Design review of the part built by this model. Coordinates are the model's own, in mm. A direction names the side the tool comes from. Coordinates: 2 decimals unless noted, no trailing zeros. Loops run counter-clockwise (first coordinate to the right, second up) from the corner with the lowest first, then second, coordinate; pieces in that order, holes last. Notation, with made-up numbers: (84.5, 1) -> (94.5, 1) arc R18 ccw to (94.5, 12) -> close; hole circle Ø4 at (-23, -24). An arc over 180 degrees is marked (long way). Use CSV: the item, a comma, the result in double quotes.
```python
from build123d import *

# Parameters (mm, degrees)
CROQUIS1_W              = 44.5
CROQUIS1_H              = 12
CROQUIS1_W_2            = 3
CROQUIS1_H_2            = 7
SALIENTE_EXTRUIR1_DEPTH = 3
EXTRUIR_L_MINA1_DEPTH   = 3


with BuildPart() as part:
    # Croquis1 → Saliente-Extruir1 (new body)
    with BuildSketch(Plane.XY):
        Polygon((-15, -12), (15, -12), (22.25, -6), (-22.25, -6), align=None)
        Rectangle(CROQUIS1_W, CROQUIS1_H)
        Polygon((9, 22), (22.25, 6), (-22.25, 6), (-9, 22), align=None)
        with Locations((23.75, 0)):
            Rectangle(CROQUIS1_W_2, CROQUIS1_H_2)
        with Locations((-23.75, 0)):
            Rectangle(CROQUIS1_W_2, CROQUIS1_H_2)
    extrude(amount=SALIENTE_EXTRUIR1_DEPTH)

    # Croquis2 → Extruir-Lámina1 (add, through all)
    with BuildSketch(Plane.XY.offset(3)):
        Polygon((10.313415418, 68.264367666), (31.70862995, 32.607243184), (0, 0), (-31.70862995, 32.607243184), (-10.313415418, 68.264367666), (-15.458313145, 71.35144191), (-39.229366975, 31.734759205), (0, -8.606356476), (39.229366975, 31.734759205), (15.458313145, 71.35144191), align=None)
    extrude(amount=-EXTRUIR_L_MINA1_DEPTH)


solid = part.part
```
Item 1: Clearance check with flat-ended pins moving along their axes: pin 1 (0.8 mm diameter, centred on y = 5.5, z = 1.5, fed in from +X); pin 2 (1 mm diameter, centred on x = -25, y = 48, fed in from -Z); pin 3 (0.9 mm diameter, centred on y = -0.5, z = 2, fed in from +X); pin 4 (0.8 mm diameter, centred on y = 4, z = 1.5, fed in from -X). State where each tip first meets the part, or that it passes through.
Checked values:
pin 1,"x = 22.25"
pin 2,"z = 0"
pin 3,"x = 25.25"
pin 4,"x = -22.25"
Item 2: Machinability: for faces 1 (the face through (24, 3.5, 1)), 2 (the face through (12.92, 69.83, 1.52)), 3 (the face through (-25.25, 0, 1)), 4 (the face through (11.81, 18.607, 1.479)), 5 (the face through (24, -3.5, 1)), which of the approach directions +Z, -Z, +X, -X, +Y, -Y give a long, thin tool a straight path to every point of the face, cutting with its end or side? Answer none if there is none.
Checked values:
face 1,"+Z, -Z, +X"
face 2,"+Z, -Z, +Y"
face 3,"+Z, -Z, -X, -Y"
face 4,"+Z, -Z"
face 5,"+Z, -Z, +X, -Y"
Item 3: Add section C-C (z = 2.55). Give the boundary of the cut face in (x, y), then the cut area to 3 significant figures.
Checked values:
outline,"(-39.23, 31.73) -> (-18.55, 10.47) -> (-22.25, 6) -> (-22.25, 3.5) -> (-25.25, 3.5) -> (-25.25, -3.5) -> (-22.25, -3.5) -> (-22.25, -6) -> (-15, -12) -> (15, -12) -> (22.25, -6) -> (22.25, -3.5) -> (25.25, -3.5) -> (25.25, 3.5) -> (22.25, 3.5) -> (22.25, 6) -> (18.55, 10.47) -> (39.23, 31.73) -> (15.46, 71.35) -> (10.31, 68.26) -> (31.71, 32.61) -> (14.7, 15.12) -> (9, 22) -> (-9, 22) -> (-14.7, 15.12) -> (-31.71, 32.61) -> (-10.31, 68.26) -> (-15.46, 71.35) -> close"
area,"2,150 mm^2"
Item 4: Add section D-D (x = 2.5). Give the boundary of the cut face in (y, z).
Checked values:
outline,"(-12, 0) -> (22, 0) -> (22, 3) -> (-12, 3) -> close"
Item 5: To check wall thickness, follow line 1 along X through (y, z) = (19.5, 1.85); line 2 along X through (y, z) = (37, 1.05); line 3 along X through (y, z) = (43.5, 0.85). State the ranges of each line that lie inside material, in increasing order.
Checked values:
line 1,"-27.33 to -18.96, -11.07 to 11.07, 18.96 to 27.33"
line 2,"-36.07 to -29.07, 29.07 to 36.07"
line 3,"-32.17 to -25.17, 25.17 to 32.17"
Item 6: Add section B-B (x = -16.5). Give the boundary of the cut face in (y, z), then the cut area to 3 significant figures.
Checked values:
outline,"(-10.76, 0) -> (16.97, 0) -> (16.97, 3) -> (-10.76, 3) -> close; (57.95, 0) -> (69.62, 0) -> (69.62, 3) -> (57.95, 3) -> close"
area,"118 mm^2"
Item 7: Add section A-A (y = 25.5). Give the boundary of the cut face in (x, z).
Checked values:
outline,"(-33.17, 0) -> (-24.8, 0) -> (-24.8, 3) -> (-33.17, 3) -> close; (24.8, 0) -> (33.17, 0) -> (33.17, 3) -> (24.8, 3) -> close"
Item 8: Draft analysis for pull direction X (two halves, no side actions). For faces 6 (the face through (-22.25, 5, 1)), 7 (the face through (-11.9, 18.5, 1.5)), 8 (the face through (0, -12, 1)), state which applies: pulls with the +X half, pulls with the -X half, needs draft (parallel to the pull), parting line crosses it, or undercut.
Checked values:
face 6,"pulls with the -X half"
face 7,"undercut"
face 8,"needs draft"
